Source: CAD feature listing. Evaluate the final solid. Frame: model axes, mm. A direction names the side the tool comes from. Give positions to 0.01 mm unless a question says otherwise; leave off trailing zeros. Order: outer loops, then holes, each group sorted by start corner. A loop starts at its lowest first (then second) coordinate and runs counter-clockwise, first axis right, second up.
from build123d import *

# Parameters (mm, degrees)
BOSS_EXTRUDE1_DEPTH = 250
SHELL1_T            = -5
SKETCH4_W           = 10
SKETCH4_H           = 5
BOSS_EXTRUDE3_DEPTH = 5
SKETCH5_R           = 1.25
CUT_EXTRUDE3_DEPTH  = 241
FILLET2_R           = 2


with BuildPart() as part:
    # Sketch1 → Boss-Extrude1 (new body)
    with BuildSketch(Plane(origin=(0, 0, 0), x_dir=(0, 0, -1), z_dir=(1, 0, 0))):
        Polygon((0, 0), (195, 0), (195, 65), (140, 120), (55, 120), (0, 65), align=None)
    extrude(amount=BOSS_EXTRUDE1_DEPTH)

    # Shell1
    shell1_openings = [part.faces().sort_by_distance(p)[0] for p in [
        (125, 0, -97.5),
    ]]
    offset(amount=SHELL1_T, openings=shell1_openings, kind=Kind.INTERSECTION)

    # Sketch4 → Boss-Extrude3 (add)
    with BuildSketch(Plane.XZ):
        with Locations((15, -192.5)):
            Rectangle(SKETCH4_W, SKETCH4_H)
        with Locations((235, -192.5)):
            Rectangle(SKETCH4_W, SKETCH4_H)
    extrude(amount=BOSS_EXTRUDE3_DEPTH)

    # Sketch5 → Cut-Extrude3 (cut, through all)
    with BuildSketch(Plane(origin=(240, 0, 0), x_dir=(0, 0, -1), z_dir=(1, 0, 0))):
        with Locations((192.5, -2.5)):
            Circle(SKETCH5_R)
    extrude(amount=-CUT_EXTRUDE3_DEPTH, mode=Mode.SUBTRACT)

    # Fillet2
    fillet2_edges = [part.edges().sort_by_distance(p)[0] for p in [
        (235, -5, -195),
        (235, -5, -190),
        (15, -5, -190),
        (15, -5, -195),
    ]]
    fillet(fillet2_edges, radius=FILLET2_R)


solid = part.part
1) Section query B-B on x = 47. Output: boundary loops of the cut face in (y, z), and give its area (3 significant figures).
Checks:
outline: (0, -195) - (65, -195) - (120, -140) - (120, -55) - (65, 0) - (0, 0) - (0, -5) - (62.93, -5) - (115, -57.07) - (115, -137.93) - (62.93, -190) - (0, -190) - close
area: 1,810 mm2
2) First-contact query: pin 1 Ø1.5 at (x, z) = (102.5, -193.5) entering from -Y; pin 2 Ø1.5 at (y, z) = (-2.5, -192.5) entering from -X; pin 3 Ø4 at (y, z) = (-3.5, -192.5) entering from -X; pin 4 Ø5 at (x, y) = (84, 100) entering from -Z. Flat tips, straight axial feed; report the tip coordinate or a pass-through.
Checks:
pin 1: stops at y = 0
pin 2: passes through
pin 3: stops at x = 10
pin 4: stops at z = -162.5
3) Pull-direction query (Z, two-part tool) for faces 1 (the face through (123, 93, -28)), 2 (the face through (5, 58, -96)), 3 (the face through (123, 120, -98)); classes: +Z half, -Z half, draft (parallel to the pull), parting line (faces both ways), or undercut.
Checks:
face 1: +Z half
face 2: undercut
face 3: draft
4) Section query D-D on y = 97. Output: boundary loops of the cut face in (x, z), and give its area (3 significant figures).
Checks:
outline: (0, -163) - (250, -163) - (250, -32) - (0, -32) - close; hole (5, -155.93) - (245, -155.93) - (245, -39.07) - (5, -39.07) - close
area: 4,700 mm2
5) Reachability of faces 4 (the face through (123, 33, 0)), 5 (the face through (123, 115, -98)) from +Z, -Z, +X, -X, +Y, -Y: full face, straight path, thin tool, end or side. Return the list, or none.
Checks:
face 4: +Z, +X, -X, +Y, -Y
face 5: -Y
6) Ray query, L1, parallel to X at y = 6, z = -105; L2, parallel to Z at x = 196, y = 40; L3, parallel to Z at x = 47, y = 89. Return the intervals inside material, ascending.
Checks:
L1: x = 0 to 5, 245 to 250
L2: z = -195 to -190, -5 to 0
L3: z = -171 to -163.93, -31.07 to -24
7) Section query A-A on y = 8. Output: boundary loops of the cut face in (x, z).
Checks:
outline: (0, -195) - (250, -195) - (250, 0) - (0, 0) - close; hole (5, -190) - (245, -190) - (245, -5) - (5, -5) - close
8) Section query C-C on z = -106.5. Output: boundary loops of the cut face in (x, y), and give its area (3 significant figures).
Checks:
outline: (0, 0) - (5, 0) - (5, 115) - (245, 115) - (245, 0) - (250, 0) - (250, 120) - (0, 120) - close
area: 2,400 mm2
